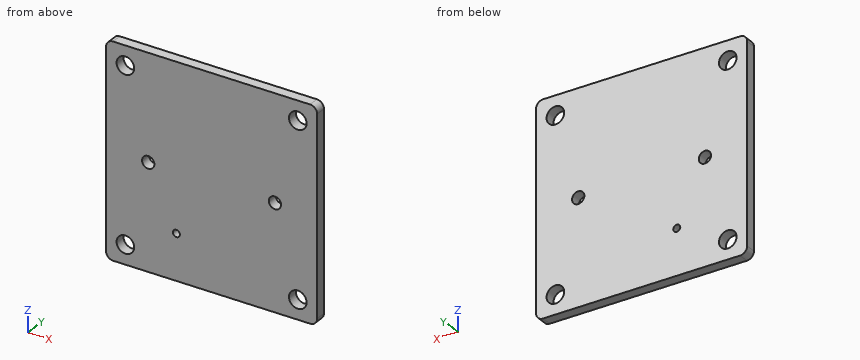
from build123d import *

# Parameters (mm, degrees)
SKETCH1_W           = 30
SKETCH1_H           = 30
SKETCH1_R           = 1.25
BOSS_EXTRUDE1_DEPTH = 1.5
FILLET1_R           = 1
SKETCH2_R           = 0.5
SKETCH2_R_2         = 0.875
CUT_EXTRUDE1_DEPTH  = 2.5


with BuildPart() as part:
    # Sketch1 → Boss-Extrude1 (new body)
    with BuildSketch(Plane(origin=(0, 0, 0), x_dir=(1, 0, 0), z_dir=(0, 1, 0))):
        Rectangle(SKETCH1_W, SKETCH1_H)
        with Locations((-12.25, 12.25)):
            Circle(SKETCH1_R, mode=Mode.SUBTRACT)
        with Locations((12.25, 12.25)):
            Circle(SKETCH1_R, mode=Mode.SUBTRACT)
        with Locations((12.25, -12.25)):
            Circle(SKETCH1_R, mode=Mode.SUBTRACT)
        with Locations((-12.25, -12.25)):
            Circle(SKETCH1_R, mode=Mode.SUBTRACT)
    extrude(amount=BOSS_EXTRUDE1_DEPTH)

    # Fillet1
    fillet1_edges = [part.edges().sort_by_distance(p)[0] for p in [
        (-15, 0.75, -15),
        (15, 0.75, -15),
        (15, 0.75, 15),
        (-15, 0.75, 15),
    ]]
    fillet(fillet1_edges, radius=FILLET1_R)

    # Sketch2 → Cut-Extrude1 (cut, through all)
    with BuildSketch(Plane(origin=(0, 1.5, 0), x_dir=(1, 0, 0), z_dir=(0, 1, 0))):
        with Locations((-5, 8.5)):
            Circle(SKETCH2_R)
        with Locations((-9, 0)):
            Circle(SKETCH2_R_2)
        with Locations((9, 0)):
            Circle(SKETCH2_R_2)
    extrude(amount=-CUT_EXTRUDE1_DEPTH, mode=Mode.SUBTRACT)


solid = part.part
Could you check a few things on this model? Use its own coordinates, in mm. Coordinates: 2 decimals unless noted, no trailing zeros. Order: outer loops, then holes, each group sorted by start corner. A loop starts at its lowest first (then second) coordinate and runs counter-clockwise, first axis right, second up. Notation, with made-up numbers: (-8, 53) - (12, 53) arc R35 ccw to (12, 88) - close; hole circle Ø1 at (-9.5, 36.5). An arc over 180 degrees is marked (long way). Answer in a Markdown table with one row per item. Add a question column.
(1) If we section it at A-A, the plane z = 12.25: Please give me the cut outline in (x, y).
(2) I need wall thicknesses on L1, parallel to X at y = 0.75, z = -12.25; L2, parallel to X at y = 0.9, z = 0 (3 decimals). Which ranges of each line are inside material? Lowest first, please.
(3) If we section it at C-C, the plane x = 12.25: Please give me the cut outline in (y, z).
(4) If we section it at B-B, the plane x = -9: Please give me the cut outline in (y, z) (3 decimals).
(5) If we section it at D-D, the plane y = 0.6: Please give me the cut outline in (x, z) (3 decimals).
(6) Will these pins go through, and if not, where does the flat tip stop? pin 1 (1.5 mm diameter, centred on x = 12.25, z = -12.25, fed in from -Y); pin 2 (3 mm diameter, centred on x = -12.25, z = 12.25, fed in from +Y).
Results are:
| question | item | result |
|---|---|---|
| 1 | outline | (-15, 0) - (-13.5, 0) - (-13.5, 1.5) - (-15, 1.5) - close; (-11, 0) - (11, 0) - (11, 1.5) - (-11, 1.5) - close; (13.5, 0) - (15, 0) - (15, 1.5) - (13.5, 1.5) - close |
| 2 | L1 | x = -15 to -13.5, -11 to 11, 13.5 to 15 |
| 2 | L2 | x = -15 to -9.875, -8.125 to 8.125, 9.875 to 15 |
| 3 | outline | (0, -15) - (1.5, -15) - (1.5, -13.5) - (0, -13.5) - close; (0, -11) - (1.5, -11) - (1.5, 11) - (0, 11) - close; (0, 13.5) - (1.5, 13.5) - (1.5, 15) - (0, 15) - close |
| 4 | outline | (0, -15) - (1.5, -15) - (1.5, -0.875) - (0, -0.875) - close; (0, 0.875) - (1.5, 0.875) - (1.5, 15) - (0, 15) - close |
| 5 | outline | (-15, -14) arc R1 ccw to (-14, -15) - (14, -15) arc R1 ccw to (15, -14) - (15, 14) arc R1 ccw to (14, 15) - (-14, 15) arc R1 ccw to (-15, 14) - close; hole circle Ø2.5 at (-12.25, -12.25); hole circle Ø2.5 at (-12.25, 12.25); hole circle Ø1.75 at (-9, 0); hole circle Ø1 at (-5, -8.5); hole circle Ø1.75 at (9, 0); hole circle Ø2.5 at (12.25, -12.25); hole circle Ø2.5 at (12.25, 12.25) |
| 6 | pin 1 | passes through |
| 6 | pin 2 | stops at y = 1.5 |
